Design review of the part built by this model. Coordinates are the model's own, in mm. Face numbers are marked on the shaded views. A direction names the side the tool comes from. Coordinates: 2 decimals unless noted, no trailing zeros. Loops run counter-clockwise (first coordinate to the right, second up) from the corner with the lowest first, then second, coordinate; pieces in that order, holes last. Notation, with made-up numbers: (-18, 89) - (18, 89) arc R11 ccw to (18, 94) - close; hole circle Ø1 at (9.25, 34). An arc over 180 degrees is marked (long way). Use one line per item in the form item = value. Start each with the question number.
(1) The part is to be moulded in two halves that separate along X. For the marked faces 1, 2 and 3, say which applies: pulls with the +X half, pulls with the -X half, needs draft (parallel to the pull), parting line crosses it, or undercut.
(2) Add section C-C (y = -6.5). State the section outline as (x, z) points.
(3) For L1, parallel to Y at x = 0, z = 8; L2, parallel to Z at x = 24, y = -9.5; L3, parallel to Z at x = 31.5, y = 7.5, list the stretches that pass through material, from the lowest coordinate up.
(4) Clearance check with flat-ended pins moving along their axes: pin 1 Ø8 at (y, z) = (-7.5, 9) entering from +X; pin 2 Ø1.5 at (y, z) = (-11, 26.5) entering from -X; pin 3 Ø6 at (x, y) = (-22.5, 5) entering from +Z; pin 4 Ø3 at (y, z) = (-16, 46) entering from -X. State where each tip first meets the part, or that it passes through.
(5) Add section D-D (x = 15). State the section outline as (y, z) points, plus the area to 3 significant figures.
(6) Add section B-B (z = 21). State the section outline as (x, y) points.
(7) Add section A-A (x = -24). State the section outline as (y, z) points, plus the area to 3 significant figures.
(8) Tool access review of the marked faces 4 and 5: name each direction out of +Z, -Z, +X, -X, +Y, -Y from which nothing blocks a thin tool from reaching the whole face with its end or side.
```python
from build123d import *

# Parameters (mm, degrees)
F2_R     = 2.54
F3_DEPTH = 7.62
F4_D     = 5.08
F4_DEPTH = 34.291
F6_D     = 5.08
F6_DEPTH = 10.16
F6_TIP   = 1.5261859723
F8_DEPTH = 3.81


with BuildPart() as f1:
    # F0 (on Front) → F1 (revolve)
    with BuildSketch(Plane.XZ):
        Polygon((27.94, 20.2932615928), (27.94, 0), (34.29, 0), (34.29, 50.8), (27.94, 50.8), align=None)
    revolve(axis=Axis((0, 0, 10.1466307964), (0, 0, 1)))

    # F2 (on face) → F3 (join)
    with BuildSketch(Plane.XY.offset(50.8)):
        with Locations((0, 31.242)):
            Circle(F2_R)
        with Locations((31.242, 0)):
            Circle(F2_R)
        with Locations((0, -31.242)):
            Circle(F2_R)
        with Locations((-31.242, 0)):
            Circle(F2_R)
    extrude(amount=F3_DEPTH)

    # F4 (through all, one way)
    with BuildSketch(Plane.XZ):
        with Locations((0, 12.7)):
            Circle(F4_D / 2)
    extrude(amount=-F4_DEPTH, mode=Mode.SUBTRACT)

    # F6
    with Locations(Plane(origin=(0, 0, 0), x_dir=(1, 0, 0), z_dir=(0, 0, -1))):
        with Locations((0, 31.242), (31.242, 0), (0, -31.242), (-31.242, 0)):
            Hole(F6_D / 2, depth=F6_DEPTH)
            with Locations((0, 0, -(F6_DEPTH + F6_TIP / 2))):  # 118° drill point
                Cone(0, F6_D / 2, F6_TIP, mode=Mode.SUBTRACT)

    # F7 (on Top) → F8 (join)
    with BuildSketch(Plane.XY):
        with BuildLine():
            Line((0, 0), (-28.1686, 0))
            ThreePointArc((-28.1686, 0), (19.9182080765, -19.9182080765), (0, 28.1686))
            Line((0, 28.1686), (0, 0))
        make_face()
    extrude(amount=F8_DEPTH)


solid = f1.part
```
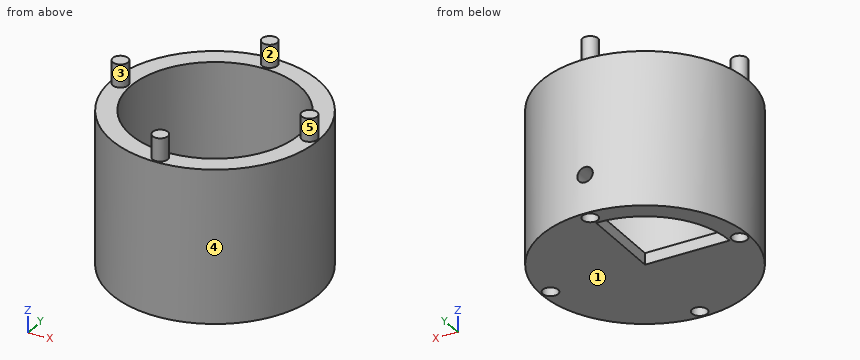
Computed values:
q1.face_1 = needs draft
q1.face_2 = parting line crosses it
q1.face_3 = undercut
q2.outline = (-33.67, 0) - (33.67, 0) - (33.67, 50.8) - (27.17, 50.8) - (27.17, 3.81) - (-27.17, 3.81) - (-27.17, 50.8) - (-33.67, 50.8) - close
q3.L1 = -34.29 to -33.78, -28.7 to -27.94, 27.94 to 28.7, 33.78 to 34.29
q3.L2 = 0 to 3.81
q3.L3 = 0 to 50.8
q4.pin_1 = 34.11
q4.pin_2 = -32.72
q4.pin_3 = through
q4.pin_4 = -31.07
q5.outline = (-30.84, 0) - (30.84, 0) - (30.84, 50.8) - (23.57, 50.8) - (23.57, 3.81) - (-23.57, 3.81) - (-23.57, 50.8) - (-30.84, 50.8) - close
q5.area = 918 mm^2
q6.outline = circle Ø68.58 at (0, 0); hole circle Ø55.88 at (0, 0)
q7.outline = (-24.49, 0) - (0, 0) - (0, 3.81) - (-14.31, 3.81) - (-14.31, 50.8) - (-24.49, 50.8) - close; (14.31, 0) - (24.49, 0) - (24.49, 50.8) - (14.31, 50.8) - close
q7.area = 1,090 mm^2
q8.face_4 = +Z, -Z
q8.face_5 = +Z
